from build123d import *

# Parameters (mm, degrees)
CROQUIS1_W              = 100
CROQUIS1_H              = 7
SALIENTE_EXTRUIR1_DEPTH = 100


with BuildPart() as part:
    # Croquis1 → Saliente-Extruir1 (new body)
    with BuildSketch(Plane.XY):
        Polygon((-40, 13.5), (-30, 3.5), (30, 3.5), (40, 13.5), align=None)
        Rectangle(CROQUIS1_W, CROQUIS1_H)
    extrude(amount=SALIENTE_EXTRUIR1_DEPTH)


solid = part.part
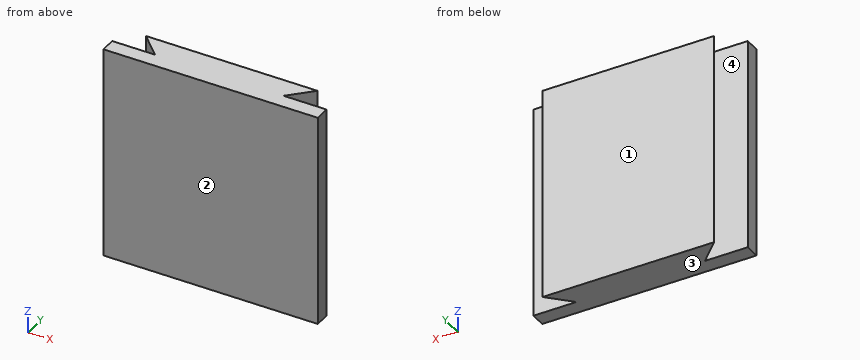
Could you check a few things on this model? Use its own coordinates, in mm. Face numbers are marked on the shaded views. Coordinates: 2 decimals unless noted, no trailing zeros. Loops run counter-clockwise (first coordinate to the right, second up) from the corner with the lowest first, then second, coordinate; pieces in that order, holes last.
1. For P1, Ø2, axis at y = 8, z = 25.5, coming from the -X side; P2, Ø1.5, axis at y = 6, z = 51, coming from the +X side; P3, Ø2, axis at y = 9, z = 17, coming from the +X side; P4, Ø22, axis at x = -42, z = 72.5, coming from the +Y side, each with a flat end and sliding along its axis, tell me the tip position at first contact or that it passes through.
2. I need wall thicknesses on L1, parallel to Y at x = 45, z = 32; L2, parallel to X at y = 11, z = 69; L3, parallel to Y at x = 38.5, z = 17.5. Which ranges of each line are inside material? Lowest first, please.
3. Imagine slicing it at B-B (z = 90.5). Please give me the cut outline in (x, y), and give its area (3 significant figures).
4. Imagine slicing it at C-C (y = 6.25). Please give me the cut outline in (x, z), and give its area (3 significant figures).
5. We'd pull the mould along Y, two halves only. Please class the marked faces 1, 2, 3 and 4: released by +Y, released by -Y, zero draft, split by the parting line, or undercut.
6. Imagine slicing it at A-A (x = 37.5). Please give me the cut outline in (y, z), and give its area (3 significant figures).
Computed values:
1. P1: stops at x = -35.5
1. P2: stops at x = 33.25
1. P3: stops at x = 36.5
1. P4: stops at y = 13.5
2. L1: y = -3.5 to 3.5
2. L2: x = -37.5 to 37.5
2. L3: y = -3.5 to 3.5, 12 to 13.5
3. outline: (-50, -3.5) - (50, -3.5) - (50, 3.5) - (30, 3.5) - (40, 13.5) - (-40, 13.5) - (-30, 3.5) - (-50, 3.5) - close
3. area: 1,400 mm2
4. outline: (-32.75, 0) - (32.75, 0) - (32.75, 100) - (-32.75, 100) - close
4. area: 6,550 mm2
5. face 1: released by +Y
5. face 2: released by -Y
5. face 3: zero draft
5. face 4: undercut
6. outline: (-3.5, 0) - (3.5, 0) - (3.5, 100) - (-3.5, 100) - close; (11, 0) - (13.5, 0) - (13.5, 100) - (11, 100) - close
6. area: 950 mm2
